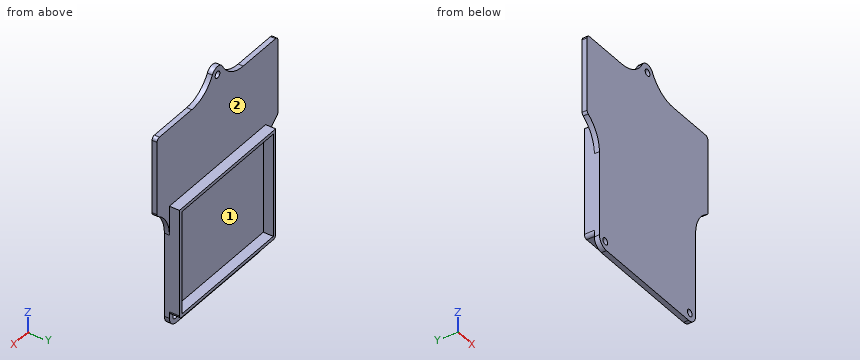
Autodesk Inventor part; units mm, degrees
ref_plane "YZ Plane" through (0, 0, 0) normal (1, 0, 0) x (0, 1, 0)
ref_plane "XZ Plane" through (0, 0, 0) normal (0, 1, 0) x (-1, 0, 0)
ref_plane "XY Plane" through (0, 0, 0) normal (0, 0, 1) x (1, 0, 0)
sketch "Sketch1" plane through (0, 0, 0) normal (0, 1, 0) x (-1, 0, 0)
  line L0 (0, 0) -> (-103, 0)
  line L1 (-103, 0) -> (-103, -121)
  line L2 (-103, -121) -> (0, -121)
  line L3 (0, -121) -> (0, 0)
  line L4 (-10.5, -121) -> (-92.5, -121)
  line L5 (-92.5, -121) -> (-92.5, -49)
  line L6 (-92.5, -49) -> (-10.5, -49)
  line L7 (-10.5, -49) -> (-10.5, -121)
  circle A0 centre (-15.5, -116) radius 2
  circle A1 centre (-87.5, -116) radius 2
  line L8 (0, -49) -> (-47, -49)
  line L9 (-47, -49) -> (-47, -2)
  line L10 (-47, -2) -> (0, -2)
  line L11 (0, -2) -> (0, -49)
  line L12 (-56, -49) -> (-103, -49)
  line L13 (-103, -49) -> (-103, -2)
  line L14 (-103, -2) -> (-56, -2)
  line L15 (-56, -2) -> (-56, -49)
  line L16 (-10.5, -49) -> (0, -49)
  line L17 (-92.5, -49) -> (-103, -49)
  circle A2 centre (-51.5, 8) radius 2
  circle A3 centre (-51.5, 8) radius 5
  line L18 (-46.5, 8) -> (-46.5, 0)
  line L19 (-46.5, 0) -> (-56.5, 0)
  line L20 (-56.5, 0) -> (-56.5, 8)
  line L21 (0, -47) -> (-103, -47)
  line L22 (-10.5, -49) -> (-10.5, -47)
  line L23 (-92.5, -49) -> (-92.5, -47)
  point P0 (0, -62)
  point P1 (-103, -62)
  point P2 (-51.5, -121)
  point P3 (-92.5, -121)
  point P4 (-10.5, -121)
  point P5 (0, -25.5)
  point P6 (-47, -25.5)
  point P7 (-56, -25.5)
  point P8 (-51.5, 0)
  point P9 (-56.5, 8)
  point P10 (-56.5, 0)
  point P11 (-46.5, 0)
  point P12 (-46.5, 8)
  dimension "d0" = 121
  dimension "d1" = 103
  dimension "d3" = 82
  dimension "d4" = 72
  dimension "d5" = 10.5
  dimension "d6" = 4
  dimension "d7" = 5
  dimension "d8" = 5
  dimension "d14" = 5
  dimension "d15" = 5
  dimension "d31" = 47
  dimension "d32" = 47
  dimension "d33" = 47
  dimension "d34" = 47
  dimension "d54" = 51.5
  dimension "d55" = 8
  dimension "d56" = 10
  dimension "d61" = 2
extrude "Extrusion1" add sketch "Sketch1" along normal blind 3 contours L3 L10 L9 L21 L15 L14 L1 L0 | L0 L20 A3 L18 | L3 L21 L9 L10 | A3 | L22 L6 L9 L21 | L9 L6 L15 L21 | L14 L15 L21 L1 | L7 L2 L5 L6 | L15 L6 L23 L21
sketch "Sketch2" plane through (0, 3, 0) normal (0, 1, 0) x (1, 0, 0)
  line L0 (0, 47) -> (47, 47)
  line L1 (47, 47) -> (47, 0)
  line L2 (47, 0) -> (0, 0)
  line L3 (0, 0) -> (0, 47)
  line L4 (0, 47) -> (0, 0)
  line L5 (0, 0) -> (103, 0)
  line L6 (56, 47) -> (103, 47)
  line L7 (103, 47) -> (103, 0)
  line L8 (103, 0) -> (56, 0)
  line L9 (56, 0) -> (56, 47)
  line L10 (103, 0) -> (103, 47)
  line L11 (92.5, 121) -> (10.5, 121)
  line L12 (10.5, 49) -> (0, 49)
  line L13 (12.5, 109) -> (90.5, 109)
  line L14 (90.5, 109) -> (90.5, 49)
  line L15 (90.5, 49) -> (12.5, 49)
  line L16 (12.5, 49) -> (12.5, 109)
  line L17 (10.5, 49) -> (10.5, 47)
  line L18 (92.5, 49) -> (92.5, 47)
  point P0 (23.5, 47)
  point P1 (105, 48)
  point P2 (0, 24.5)
  point P3 (10.5, 121)
  point P4 (56, 23.5)
  point P5 (47, 23.5)
  point P6 (0, 104.7)
  point P7 (105, 104.7)
  point P8 (103, 49)
  point P9 (90.5, 79)
  point P10 (12.5, 79)
  dimension "d21" = 47
  dimension "d22" = 47
  dimension "d26" = 47
  dimension "d38" = 2
  dimension "d39" = 78
  dimension "d40" = 60
  dimension "d43" = 12.5
sketch "Sketch3" plane through (0, 3, 0) normal (0, 1, 0) x (1, 0, 0)
  line L0 (10.5, 113) -> (92.5, 113)
  line L1 (92.5, 113) -> (92.5, 47)
  line L2 (92.5, 47) -> (10.5, 47)
  line L3 (10.5, 47) -> (10.5, 113)
  line L4 (12.5, 111) -> (90.5, 111)
  line L5 (90.5, 111) -> (90.5, 49)
  line L6 (90.5, 49) -> (12.5, 49)
  line L7 (12.5, 49) -> (12.5, 111)
  line L8 (0, 47) -> (0, 0)
  line L9 (0, 0) -> (103, 0)
  point P0 (0, 49)
  dimension "d44" = 78
  dimension "d45" = 62
  dimension "d46" = 12.5
  dimension "d47" = 49
  dimension "d48" = 82
  dimension "d49" = 2
  dimension "d51" = 66
  dimension "d52" = 2
fillet "Fillet1" radius 20 2 edges at (56.5, 1.5, 0) (46.5, 1.5, 0)
extrude "Extrusion2" add sketch "Sketch3" along normal blind 6
fillet "Fillet3" radius 20 2 edges at (92.5, 1.5, -47) (10.5, 1.5, -47)
fillet "Fillet4" radius 6 2 edges at (92.5, 1.5, -121) (10.5, 1.5, -121)
fillet "Fillet5" radius 2 6 edges at (0, 1.5, 0) (103, 1.5, 0) (0, 1.5, -47) (103, 1.5, -47) (92.5, 6, -113) (10.5, 6, -113)
equation "\"d0\" = d34 + d37 + d4"
equation "\"d1\" = 2 * d47 + d36"
equation "\"d5\" = -0.5 * d3 + 0.5 * d1"
equation "\"d54\" = 0.5 * d1"
equation "\"d38\" = d37"
equation "\"d43\" = -0.5 * d39 + 0.5 * d1"
equation "\"d44\" = d39"
equation "\"d46\" = d43"
equation "\"d47\" = d38 + d21"
equation "\"d48\" = d3"
equation "\"d2\" = 0.5 * d0"
properties part number "baseCarrito2"
Verification items for the finished model (mm, model axes). Face numbers are marked on the shaded views. Give positions to 0.01 mm unless a question says otherwise; leave off trailing zeros. Order: outer loops, then holes, each group sorted by start corner. A loop starts at its lowest first (then second) coordinate and runs counter-clockwise, first axis right, second up. Notation, with made-up numbers: (-10.75, 37.5) -> (26.25, 37.5) arc R28 cw to (26.25, 70.5) -> close; hole circle Ø8 at (72.5, -20). An arc over 180 degrees is marked (long way). One line per item, written item: value.
(1) Gauge pin test, flat ends, axial feed: pin 1 (1.8 mm diameter, centred on x = 54.5, y = 5.5, fed in from +Z); pin 2 (5 mm diameter, centred on x = 61, y = 6, fed in from -Z); pin 3 (0.9 mm diameter, centred on x = 93.5, y = 2, fed in from +Z). Record the tip position at first contact, or that the pin passes through.
Final values:
pin 1: z = -47
pin 2: z = -113
pin 3: z = 0
(2) Sectioned sample at D-D on x = 82.5. Record the cut outline in (y, z), then the cut area to 3 significant figures.
Final values:
outline: (0, -121) -> (3, -121) -> (3, -113) -> (9, -113) -> (9, -111) -> (3, -111) -> (3, -49) -> (9, -49) -> (9, -47) -> (3, -47) -> (3, 0) -> (0, 0) -> close
area: 387 mm^2
(3) Sectioned sample at A-A on x = 51.5. Record the cut outline in (y, z).
Final values:
outline: (0, -121) -> (3, -121) -> (3, -113) -> (9, -113) -> (9, -111) -> (3, -111) -> (3, -49) -> (9, -49) -> (9, -47) -> (3, -47) -> (3, 6) -> (0, 6) -> close; (0, 10) -> (3, 10) -> (3, 13) -> (0, 13) -> close
(4) Sectioned sample at C-C on z = -109. Record the cut outline in (x, y).
Final values:
outline: (10.5, 0) -> (92.5, 0) -> (92.5, 9) -> (90.5, 9) -> (90.5, 3) -> (12.5, 3) -> (12.5, 9) -> (10.5, 9) -> close
(5) Sectioned sample at B-B on y = 5.25. Record the cut outline in (x, z).
Final values:
outline: (10.5, -111) arc R2 ccw to (12.5, -113) -> (90.5, -113) arc R2 ccw to (92.5, -111) -> (92.5, -47) -> (10.5, -47) -> close; hole (12.5, -111) -> (90.5, -111) -> (90.5, -49) -> (12.5, -49) -> close
(6) Draft check along X on the marked faces 1 and 2. Enter one of: pulls with the +X half, pulls with the -X half, needs draft (parallel to the pull), parting line crosses it, or undercut.
Final values:
face 1: undercut
face 2: needs draft
(7) Scan lines: line 1 along X through (y, z) = (4, -102); line 2 along Z through (x, y) = (14.5, 5); line 3 along Z through (x, y) = (51.5, 1.8). Record each from-to range of solid material in increasing order. Write a range as [from, to].
Final values:
line 1: [10.5, 12.5], [90.5, 92.5]
line 2: [-113, -111], [-49, -47]
line 3: [-121, 6], [10, 13]
